from build123d import *

# Parameters (mm, degrees)
F0_W     = 76.2886069715
F0_H     = 38.1443016231
F1_DEPTH = 76.2
F2_R     = 38.09999
F4_D     = 58.42
F4_DEPTH = 12.7
F4_TIP   = 17.5511386818
F5_R     = 38.09999
F6_R     = 12.7378189323
F7_DEPTH = 25.4


# Not quite as in the source:
# - a fillet or chamfer is up to 0.001 mm smaller than in the source, because OpenCascade refuses the exact size


with BuildPart() as f1:
    # F0 (on Top) → F1 (new body)
    with BuildSketch(Plane.XY):
        with Locations((-1.0466407984, 2.4421662092)):
            Rectangle(F0_W, F0_H)
    extrude(amount=F1_DEPTH)

    # F2 (radius 38.1 in the source; OpenCascade refuses exactly that, so slightly less here)
    f2_edges = [f1.edges().sort_by_distance(p)[0] for p in [
        (-39.190944, 2.442166, 76.2),
        (-39.190944, 2.442166, 0),
        (37.097663, 2.442166, 76.2),
        (37.097663, 2.442166, 0),
    ]]
    fillet(f2_edges, radius=F2_R)

    # F4
    with Locations(Plane.XZ.offset(16.6299846023)):
        with Locations((-1.0909442842, 38.1)):
            Hole(F4_D / 2, depth=F4_DEPTH)
            with Locations((0, 0, -(F4_DEPTH + F4_TIP / 2))):  # 118° drill point
                Cone(0, F4_D / 2, F4_TIP, mode=Mode.SUBTRACT)

    # F5 (radius 38.1 in the source; OpenCascade refuses exactly that, so slightly less here)
    f5_edges = [f1.edges().sort_by_distance(p)[0] for p in [
        (-28.031716, 21.514317, 11.159229),
        (25.938434, 21.514317, 11.159229),
    ]]
    fillet(f5_edges, radius=F5_R)

    # F6 (on Front) → F7 (join)
    with BuildSketch(Plane.XZ):
        with Locations((-1.6050767154, 35.1008698344)):
            Circle(F6_R)
    extrude(amount=-F7_DEPTH)


solid = f1.part
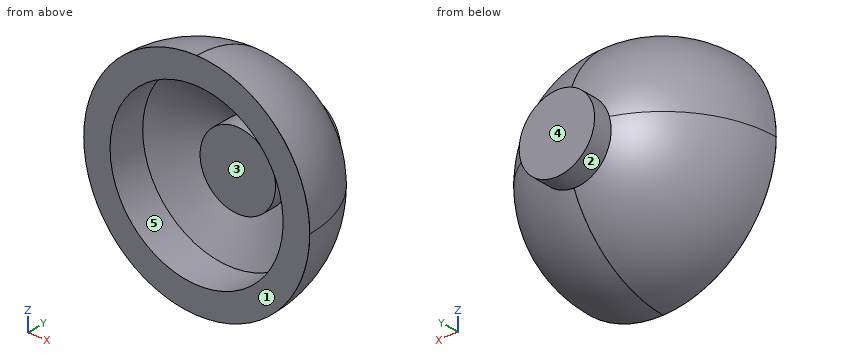
Part model, mm, in its own coordinate system. Face numbers are marked on the shaded views. A direction names the side the tool comes from. Give positions to 0.01 mm unless a question says otherwise; leave off trailing zeros. Order: outer loops, then holes, each group sorted by start corner. A loop starts at its lowest first (then second) coordinate and runs counter-clockwise, first axis right, second up. Notation, with made-up numbers: (76, -6.5) -> (104, -6.5) arc R22 cw to (104, 24.5) -> close; hole circle Ø9 at (12, 8). An arc over 180 degrees is marked (long way). Use one line per item in the form item = value.
(1) Tool access for the marked faces 4 and 5: list every direction of +Z, -Z, +X, -X, +Y, -Y with a clear straight run to the whole face (end or side of a thin tool).
Solution:
face_4 = +Z, -Z, +X, -X, +Y
face_5 = -Y
(2) Flat gauge pins, fed straight in: P1, Ø10, axis at x = -8, y = -3.5, coming from the +Z side; P2, Ø1, axis at x = 14.5, y = 7, coming from the +Z side; P3, Ø10, axis at x = -15.5, y = 10.5, coming from the -Z side. Where does each tip first touch, or does it go through?
Solution:
P1 = 74.92
P2 = 64.23
P3 = 9.95
(3) Saw through at C-C (y = 23.5). Write the cut outline in (x, z), then the cut area to 3 significant figures.
Solution:
outline = circle Ø25.48 at (-1.61, 35.1)
area = 510 mm²
(4) Drill centre lines: line 1 (Z direction, x = -4.5, y = -13); line 2 (X direction, y = -0.5, z = 35); line 3 (Z direction, x = 14, y = -1). Where is each one in solid material? Low to high. Write a range as from..to.
Solution:
line_1 = 0.32..9.09, 67.11..75.88
line_2 = -35.49..-24.39, 22.21..33.4
line_3 = 6.74..19.01, 57.19..69.46
(5) Pull direction Z, two halves, no side cores. Call the marked faces 1, 2 and 3: +Z half, -Z half, draft (parallel to the pull), parting line (faces both ways), or undercut.
Solution:
face_1 = draft
face_2 = parting line
face_3 = undercut
